```python
from build123d import *

# Parameters (mm, degrees)
SKETCH1_R           = 54.524863565
SKETCH1_R_2         = 41
BOSS_EXTRUDE1_DEPTH = 5
SKETCH2_R           = 45.441734001
SKETCH2_R_2         = 38.435146228
BOSS_EXTRUDE2_DEPTH = 5
FILLET1_R           = 5


with BuildPart() as part:
    # Sketch1 → Boss-Extrude1 (new body)
    with BuildSketch(Plane.XY):
        Circle(SKETCH1_R)
        Circle(SKETCH1_R_2, mode=Mode.SUBTRACT)
    extrude(amount=BOSS_EXTRUDE1_DEPTH)

    # Sketch2 → Boss-Extrude2 (add)
    with BuildSketch(Plane.XY.offset(5)):
        Circle(SKETCH2_R)
        Circle(SKETCH2_R_2, mode=Mode.SUBTRACT)
    extrude(amount=BOSS_EXTRUDE2_DEPTH)

    # Fillet1
    fillet1_edges = [part.edges().sort_by_distance(p)[0] for p in [
        (-45.441734001, 0, 5),
    ]]
    fillet(fillet1_edges, radius=FILLET1_R - 0.0001)  # a hair under: the kernel refuses the full size


solid = part.part
```
Work out the finished part from the listing and answer in its coordinate system (mm). A direction names the side the tool comes from. Give positions to 0.01 mm unless a question says otherwise; leave off trailing zeros. Write each loop counter-clockwise with the first axis right and the second up, starting at its lowest first coordinate (ties: lowest second). Pieces come first, ordered by that corner, then holes.
(1) Flat-ended cylindrical pins translate along their axes: pin 1 Ø5 at (x, z) = (-38.5, 5.5) entering from +Y; pin 2 Ø5 at (x, z) = (-30, 6.5) entering from +Y; pin 3 Ø5 at (y, z) = (-34.5, 3) entering from +X. Find the tip coordinate at first contact, or state that the pin passes through.
Final values:
pin 1: stops at y = 40.91
pin 2: stops at y = 46.79
pin 3: stops at x = 44.15
(2) The mould has two halves that part along X. Classify faces 3 (the cylindrical face through (17.735, -34.099, 7.465)), 4 (the cylindrical face through (-9, -40, 2)), 5 (the flat face through (16, -48, 5)), 6 (the cylindrical face through (-43.269, -33.178, 2.465)): pulls with the +X half, pulls with the -X half, needs draft (parallel to the pull), parting line crosses it, or undercut.
Final values:
face 3: undercut
face 4: undercut
face 5: needs draft
face 6: parting line crosses it
(3) Which of the six approach directions +Z, -Z, +X, -X, +Y, -Y give full straight-line access (tool end or side, diameter ignored) to faces 1 (the flat face through (-37, -12, 5)), 2 (the flat face through (-37.2, 10.3, 10))?
Final values:
face 1: -Z
face 2: +Z, +X, -X, +Y, -Y
(4) Straight lines are drawn through the part: line 1 (Y direction, x = 0, z = 2.6); line 2 (Z direction, x = 15, y = -48.5); line 3 (Y direction, x = 12, z = 8). For each, find the intervals that lie inside material, in ascending order.
Final values:
line 1: y = -54.52 to -41, 41 to 54.52
line 2: z = 0 to 5
line 3: y = -44.26 to -36.51, 36.51 to 44.26
(5) The part is cut by section C-C on z = 3.5. Write down the section's boundary in (x, y), plus the area to 3 significant figures.
Final values:
outline: circle Ø109.05 at (0, 0); hole circle Ø82 at (0, 0)
area: 4,060 mm2
